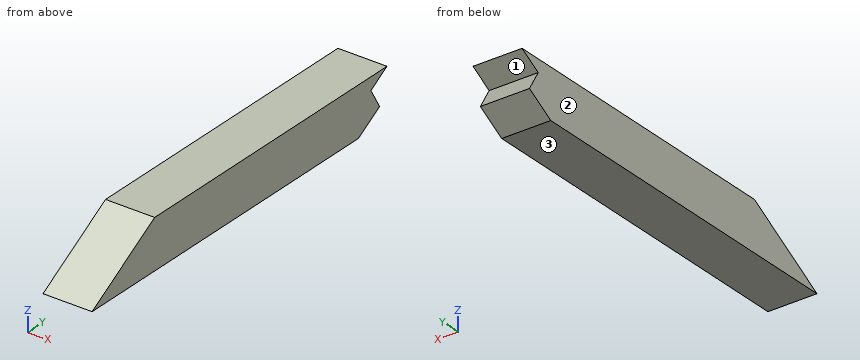
```python
from build123d import *

# Parameters (mm, degrees)
F0_W     = 190.5
F0_H     = 190.5
F1_DEPTH = 1524
F3_DEPTH = 190.501
F5_DEPTH = 190.501


with BuildPart() as f1:
    # F0 (on Front) → F1 (new body)
    with BuildSketch(Plane.XZ):
        with Locations((95.25, 95.25)):
            Rectangle(F0_W, F0_H)
    extrude(amount=F1_DEPTH)

    # F2 (on face) → F3 (cut, through all)
    with BuildSketch(Plane.YZ.offset(190.5)):
        Polygon((-1524, 190.5), (-1524, 0), (-1200.727273, 190.5), align=None)
        Polygon((-83.324024, 141.398343), (0, 0), (0, 190.5), align=None)
    extrude(amount=-F3_DEPTH, mode=Mode.SUBTRACT)

    # F4 (on face) → F5 (cut, through all)
    with BuildSketch(Plane.YZ.offset(190.5)):
        Polygon((0, 0), (-38.190178, 64.807574), (-148.166667, 0), align=None)
    extrude(amount=-F5_DEPTH, mode=Mode.SUBTRACT)


solid = f1.part
```
Build history of the part. All positions in model axes, mm. Face numbers are marked on the shaded views. Give positions to 0.01 mm unless a question says otherwise; leave off trailing zeros. Loops run counter-clockwise (first coordinate to the right, second up) from the corner with the lowest first, then second, coordinate; pieces in that order, holes last.
1) Drop flat-ended pins along their axis: P1, Ø2, axis at x = 79, z = 70.5, coming from the -Y side; P2, Ø5, axis at x = 170, z = 124, coming from the -Y side; P3, Ø1.5, axis at x = 39.5, z = 31, coming from the -Y side. Give the stop position or say it passes through.
Values follow:
P1: stops at y = -1406.06
P2: stops at y = -1317.82
P3: stops at y = -1472.67
2) Two-plate mould, pull along Z, no slides. Class the marked faces 1, 2 and 3: released by +Z, released by -Z, zero draft, split by the parting line, or undercut.
Values follow:
face 1: undercut
face 2: zero draft
face 3: released by -Z
3) Band-saw the part on A-A on x = 101.5. List the corners of the cut face in (y, z), then the cut area to 3 significant figures.
Values follow:
outline: (-1524, 0) - (-148.17, 0) - (-38.19, 64.81) - (-83.32, 141.4) - (0, 190.5) - (-1200.73, 190.5) - close
area: 247,000 mm2
4) Band-saw the part on C-C on y = -1346.5. List the corners of the cut face in (x, z), then the cut area to 3 significant figures.
Values follow:
outline: (0, 0) - (190.5, 0) - (190.5, 104.6) - (0, 104.6) - close
area: 19,900 mm2
5) Band-saw the part on B-B on z = 110. List the corners of the cut face in (x, y), then the cut area to 3 significant figures.
Values follow:
outline: (0, -1337.33) - (190.5, -1337.33) - (190.5, -64.82) - (0, -64.82) - close
area: 242,000 mm2
6) Probe line 1 along Z through (x, y) = (105.5, -1389.5); line 2 along Y through (x, z) = (168.5, 94.5); line 3 along Y through (x, z) = (138, 145.5). List the from-to ranges inside material, lowest first.
Values follow:
line 1: z = 0 to 79.26
line 2: y = -1363.64 to -55.69
line 3: y = -1277.09 to -76.36
